from build123d import *

# Parameters (mm, degrees)
F1_DEPTH = 25.4


with BuildPart() as f1:
    # F0 (on Top) → F1 (new body)
    with BuildSketch(Plane.XY):
        with BuildLine():
            ThreePointArc((0, 13.190946), (13.190946, 0), (0, -13.190946))
            Line((0, -13.190946), (-9.774976, -13.190946))
            Line((-9.774976, -13.190946), (-9.774976, -20.837533))
            Line((-9.774976, -20.837533), (0, -20.837533))
            ThreePointArc((0, -20.837533), (20.837533, 0), (0, 20.837533))
            ThreePointArc((0, 20.837533), (-12.708639, 33.546172), (0, 46.254811))
            Line((0, 46.254811), (9.050903, 46.254811))
            Line((9.050903, 46.254811), (9.050903, 53.901398))
            Line((9.050903, 53.901398), (0, 53.901398))
            ThreePointArc((0, 53.901398), (-20.355226, 33.546172), (0, 13.190946))
        make_face()
    extrude(amount=F1_DEPTH)


solid = f1.part
The listing builds one solid part. Answer for the finished solid, in the listing's coordinates (mm). A direction names the side the tool comes from. Round coordinates to 2 decimals unless told otherwise and drop trailing zeros. Order: outer loops, then holes, each group sorted by start corner. A loop starts at its lowest first (then second) coordinate and runs counter-clockwise, first axis right, second up. Notation, with made-up numbers: (80.5, -11) -> (117.5, -11) arc R27 ccw to (117.5, 22) -> close; hole circle Ø5 at (61.25, 54). An arc over 180 degrees is marked (long way). Write each question's results on one line, items separated by ' | '. Start each with the question number.
Q1. Straight lines are drawn through the part: probe 1 along Y at (x, z) = (7, 20.5); probe 2 along Y at (x, z) = (-8, 22.75); probe 3 along X at (y, z) = (33, 14). For each, find the intervals that lie inside material, in ascending order. Write a range as from..to.
Q2. The mould has two halves that part along Y. Classify faces 1 (the flat face through (-5, -13.191, 13)), 2 (the flat face through (5, 53.901, 13)), 3 (the cylindrical face through (-12.706, 33.267, 12.522)), 4 (the flat face through (9.051, 50, 13)): pulls with the +Y half, pulls with the -Y half, needs draft (parallel to the pull), parting line crosses it, or undercut.
Q3. Find section C-C (x = 10). Determine the outline of the cut face in (y, z).
Q4. Each of these flat-tipped pins is pushed along its axis until it touches: pin 1 (2 mm diameter, centred on x = 16.5, z = 10.5, fed in from +Y); pin 2 (4 mm diameter, centred on y = -17, z = 16, fed in from -X) (3 decimals); pin 3 (12 mm diameter, centred on y = -1.5, z = 8, fed in from +X). Where does it stop, or does it pass through?
Q5. Find section D-D (x = -5.5). Determine the outline of the cut face in (y, z).
Q6. Find section B-B (y = 0). Determine the outline of the cut face in (x, z), then the cut area to 3 significant figures.
Q7. Which of the six approach directions +Z, -Z, +X, -X, +Y, -Y give full straight-line access (tool end or side, diameter ignored) to faces 5 (the flat face through (4, 46.255, 13)), 6 (the cylindrical face through (-20.35, 33.99, 12.52)), 7 (the flat face through (-9.775, -17, 13))?
Q8. Find section A-A (x = -1). Determine the outline of the cut face in (y, z), then the cut area to 3 significant figures.
Worked answers:
1) probe 1: y = -19.63..-11.18, 11.18..19.63, 46.25..53.9 | probe 2: y = -20.84..-13.19, 14.83..23.67, 43.42..52.26 | probe 3: x = -20.35..-12.7
2) face 1: undercut | face 2: pulls with the +Y half | face 3: undercut | face 4: needs draft
3) outline: (-18.28, 0) -> (-8.6, 0) -> (-8.6, 25.4) -> (-18.28, 25.4) -> close; (8.6, 0) -> (18.28, 0) -> (18.28, 25.4) -> (8.6, 25.4) -> close
4) pin 1: stops at y = 13.93 | pin 2: stops at x = -9.775 | pin 3: stops at x = 20.84
5) outline: (-20.84, 0) -> (-13.19, 0) -> (-13.19, 25.4) -> (-20.84, 25.4) -> close; (13.95, 0) -> (22.09, 0) -> (22.09, 25.4) -> (13.95, 25.4) -> close; (45, 0) -> (53.14, 0) -> (53.14, 25.4) -> (45, 25.4) -> close
6) outline: (13.19, 0) -> (20.84, 0) -> (20.84, 25.4) -> (13.19, 25.4) -> close | area: 194 mm2
7) face 5: +Z, -Z, +X | face 6: +Z, -Z, -X | face 7: +Z, -Z, -X, -Y
8) outline: (-20.84, 0) -> (-13.19, 0) -> (-13.19, 25.4) -> (-20.84, 25.4) -> close; (13.22, 0) -> (20.88, 0) -> (20.88, 25.4) -> (13.22, 25.4) -> close; (46.22, 0) -> (53.88, 0) -> (53.88, 25.4) -> (46.22, 25.4) -> close | area: 583 mm2
